Geometry check sheet. Reference: the model listing, model coordinates, mm. A direction names the side the tool comes from. Round coordinates to 2 decimals unless told otherwise and drop trailing zeros. Loops run counter-clockwise (first coordinate to the right, second up) from the corner with the lowest first, then second, coordinate; pieces in that order, holes last. Notation, with made-up numbers: (-3.75, 38) - (27.25, 38) arc R20 ccw to (27.25, 51) - close; hole circle Ø8 at (-2.5, 29). An arc over 180 degrees is marked (long way). Write item = value, one per line.
```python
from build123d import *

# Parameters (mm, degrees)
SKETCH1_W           = 156
SKETCH1_H           = 196
BASE_FLANGE1_DEPTH  = 0.5
EDGE_FLANGE1_DEPTH  = 196
EDGE_FLANGE2_DEPTH  = 156
EDGE_FLANGE3_DEPTH  = 196
EDGE_FLANGE4_DEPTH  = 156
SKETCH14_R          = 3
CUT_EXTRUDE1_DEPTH  = 2
CUT_EXTRUDE2_START  = -0.5
CUT_EXTRUDE2_DEPTH  = 0.5
CUT_EXTRUDE7_START  = -0.5
CUT_EXTRUDE7_DEPTH  = 0.5
SKETCH18_R          = 2
CUT_EXTRUDE8_DEPTH  = 254.83311453
SKETCH19_R          = 2
CUT_EXTRUDE9_DEPTH  = 255.06938035
SKETCH20_R          = 4
CUT_EXTRUDE10_DEPTH = 5
CUT_EXTRUDE11_START = -5
SKETCH21_R          = 4
CUT_EXTRUDE11_DEPTH = 5
SKETCH22_R          = 4
CUT_EXTRUDE12_DEPTH = 5
CUT_EXTRUDE13_START = -5
SKETCH23_R          = 4
CUT_EXTRUDE13_DEPTH = 5
SKETCH24_R          = 10
CUT_EXTRUDE14_DEPTH = 1
SKETCH25_R          = 2
CUT_EXTRUDE15_DEPTH = 2


# Read off the part's stored shape, not the designer's step: Cut-Extrude2, Cut-Extrude7
# Sheet-metal steps are written as plain solids
with BuildPart() as part:
    # Sketch1 → Base-Flange1 (new body)
    with BuildSketch(Plane(origin=(0, 0, 0), x_dir=(1, 0, 0), z_dir=(0, 1, 0))):
        with Locations((78, -98)):
            Rectangle(SKETCH1_W, SKETCH1_H)
    extrude(amount=-BASE_FLANGE1_DEPTH)

    # Edge-Flange1 section (across the edge) → Edge-Flange1 (add)
    with BuildSketch(Plane(origin=(-1, 0, 0), x_dir=(1, 0, 0), z_dir=(0, 0, 1))):
        with BuildLine():
            Line((-0.5, 1), (-0.5, 12))
            Line((-0.5, 12), (0, 12))
            Line((0, 12), (0, 1))
            ThreePointArc((0, 1), (0.292893219, 0.292893219), (1, 0))
            Line((1, 0), (1, -0.5))
            ThreePointArc((1, -0.5), (-0.060660172, -0.060660172), (-0.5, 1))
        make_face()
    extrude(amount=EDGE_FLANGE1_DEPTH)

    # Edge-Flange2 section (across the edge) → Edge-Flange2 (add)
    with BuildSketch(Plane(origin=(0, 0, 197), x_dir=(0, 0, -1), z_dir=(1, 0, 0))):
        with BuildLine():
            Line((-0.5, 1), (-0.5, 12))
            Line((-0.5, 12), (0, 12))
            Line((0, 12), (0, 1))
            ThreePointArc((0, 1), (0.292893219, 0.292893219), (1, 0))
            Line((1, 0), (1, -0.5))
            ThreePointArc((1, -0.5), (-0.060660172, -0.060660172), (-0.5, 1))
        make_face()
    extrude(amount=EDGE_FLANGE2_DEPTH)

    # Edge-Flange3 section (across the edge) → Edge-Flange3 (add)
    with BuildSketch(Plane(origin=(157, 0, 196), x_dir=(-1, 0, 0), z_dir=(0, 0, -1))):
        with BuildLine():
            Line((-0.5, 1), (-0.5, 12))
            Line((-0.5, 12), (0, 12))
            Line((0, 12), (0, 1))
            ThreePointArc((0, 1), (0.292893219, 0.292893219), (1, 0))
            Line((1, 0), (1, -0.5))
            ThreePointArc((1, -0.5), (-0.060660172, -0.060660172), (-0.5, 1))
        make_face()
    extrude(amount=EDGE_FLANGE3_DEPTH)

    # Edge-Flange4 section (across the edge) → Edge-Flange4 (add)
    with BuildSketch(Plane(origin=(156, 0, -1), x_dir=(0, 0, 1), z_dir=(-1, 0, 0))):
        with BuildLine():
            Line((-0.5, 1), (-0.5, 12))
            Line((-0.5, 12), (0, 12))
            Line((0, 12), (0, 1))
            ThreePointArc((0, 1), (0.292893219, 0.292893219), (1, 0))
            Line((1, 0), (1, -0.5))
            ThreePointArc((1, -0.5), (-0.060660172, -0.060660172), (-0.5, 1))
        make_face()
    extrude(amount=EDGE_FLANGE4_DEPTH)

    # Sketch14 → Cut-Extrude1 (cut)
    with BuildSketch(Plane.XY.offset(197.5)):
        with Locations((88.5, 5.312571767)):
            Circle(SKETCH14_R)
        with Locations((67.5, 5.312571767)):
            Circle(SKETCH14_R)
    extrude(amount=-CUT_EXTRUDE1_DEPTH, mode=Mode.SUBTRACT)

    # Cut-Extrude2 outline → Cut-Extrude2 (cut)
    with BuildSketch(Plane.ZY.offset(1.5).offset(CUT_EXTRUDE2_START)):
        with BuildLine():
            ThreePointArc((7.181368129, 12), (14.44892966, 4.034634629), (24.795691895, 1))
            add(Edge.make_bspline(
                [(24.795691895, 1), (24.960369193, 1), (25.12504649, 1), (25.289723788, 1)],
                knots=[0, 0, 0, 0, 1, 1, 1, 1], degree=3))
            ThreePointArc((25.289723788, 1), (35.636486024, 4.034634629), (42.904047554, 12))
            Line((42.904047554, 12), (7.181368129, 12))
        make_face()
        with BuildLine():
            Line((189.110571099, 12), (153.389428901, 12))
            ThreePointArc((153.389428901, 12), (171.25, 1), (189.110571099, 12))
        make_face()
    extrude(amount=CUT_EXTRUDE2_DEPTH, mode=Mode.SUBTRACT)

    # Cut-Extrude7 outline → Cut-Extrude7 (cut)
    with BuildSketch(Plane(origin=(157.5, 0, 0), x_dir=(0, 0, -1), z_dir=(1, 0, 0)).offset(CUT_EXTRUDE7_START)):
        with BuildLine():
            ThreePointArc((-189.110571099, 12), (-171.25, 1), (-153.389428901, 12))
            Line((-153.389428901, 12), (-189.110571099, 12))
        make_face()
        with BuildLine():
            add(Edge.make_bspline(
                [(-24.795691895, 1), (-24.960369193, 1), (-25.12504649, 1), (-25.289723788, 1)],
                knots=[0, 0, 0, 0, 1, 1, 1, 1], degree=3))
            ThreePointArc((-24.795691895, 1), (-14.44892966, 4.034634629), (-7.181368129, 12))
            Line((-7.181368129, 12), (-42.904047554, 12))
            ThreePointArc((-42.904047554, 12), (-35.636486024, 4.034634629), (-25.289723788, 1))
        make_face()
    extrude(amount=CUT_EXTRUDE7_DEPTH, mode=Mode.SUBTRACT)

    # Sketch18 → Cut-Extrude8 (cut, through all)
    with BuildSketch(Plane(origin=(157.5, 0, 0), x_dir=(0, 0, -1), z_dir=(1, 0, 0))):
        with Locations(Location((-98.146856175, 5.118141575, 0), (0, 0, 90))):
            Circle(SKETCH18_R)
    extrude(amount=-CUT_EXTRUDE8_DEPTH, mode=Mode.SUBTRACT)

    # Sketch19 → Cut-Extrude9 (cut, through all)
    with BuildSketch(Plane.XY.offset(197.5)):
        with Locations((27.98454493, 5.280354993)):
            Circle(SKETCH19_R)
        with Locations(Location((128.01545507, 5.280354993, 0), (0, 0, 180))):
            Circle(SKETCH19_R)
    extrude(amount=-CUT_EXTRUDE9_DEPTH, mode=Mode.SUBTRACT)

    # Sketch20 → Cut-Extrude10 (cut)
    with BuildSketch(Plane(origin=(157.5, 0, 0), x_dir=(0, 0, -1), z_dir=(1, 0, 0))):
        with Locations(Location((-88.146856175, 5.118141575, 0), (0, 0, 90))):
            Circle(SKETCH20_R)
        with Locations(Location((-108.146856175, 5.118141575, 0), (0, 0, 90))):
            Circle(SKETCH20_R)
    extrude(amount=-CUT_EXTRUDE10_DEPTH, mode=Mode.SUBTRACT)

    # Sketch21 → Cut-Extrude11 (cut)
    with BuildSketch(Plane.ZY.offset(1.5).offset(CUT_EXTRUDE11_START)):
        with Locations(Location((88.146856175, 5.118141575, 0), (0, 0, 90))):
            Circle(SKETCH21_R)
        with Locations(Location((108.146856175, 5.118141575, 0), (0, 0, 90))):
            Circle(SKETCH21_R)
    extrude(amount=CUT_EXTRUDE11_DEPTH, mode=Mode.SUBTRACT)

    # Sketch22 → Cut-Extrude12 (cut)
    with BuildSketch(Plane.XY.offset(197.5)):
        with Locations((138, 5.25)):
            Circle(SKETCH22_R)
        with Locations((118, 5.25)):
            Circle(SKETCH22_R)
        with Locations((38, 5.25)):
            Circle(SKETCH22_R)
        with Locations((18, 5.25)):
            Circle(SKETCH22_R)
    extrude(amount=-CUT_EXTRUDE12_DEPTH, mode=Mode.SUBTRACT)

    # Sketch23 → Cut-Extrude13 (cut)
    with BuildSketch(Plane(origin=(0, 0, -1.5), x_dir=(-1, 0, 0), z_dir=(0, 0, -1)).offset(CUT_EXTRUDE13_START)):
        with Locations(Location((-18, 5.25, 0), (0, 0, 180))):
            Circle(SKETCH23_R)
        with Locations(Location((-38, 5.25, 0), (0, 0, 180))):
            Circle(SKETCH23_R)
        with Locations(Location((-118, 5.25, 0), (0, 0, 180))):
            Circle(SKETCH23_R)
        with Locations(Location((-138, 5.25, 0), (0, 0, 180))):
            Circle(SKETCH23_R)
    extrude(amount=CUT_EXTRUDE13_DEPTH, mode=Mode.SUBTRACT)

    # Sketch24 → Cut-Extrude14 (cut)
    with BuildSketch(Plane.XY.offset(197.5)):
        with Locations((78, 17.812571767)):
            Circle(SKETCH24_R)
    extrude(amount=-CUT_EXTRUDE14_DEPTH, mode=Mode.SUBTRACT)

    # Sketch25 → Cut-Extrude15 (cut)
    with BuildSketch(Plane.XZ.offset(0.5)):
        with Locations(Location((78, 182.993325715, 0), (0, 0, 270))):
            Circle(SKETCH25_R)
    extrude(amount=-CUT_EXTRUDE15_DEPTH, mode=Mode.SUBTRACT)


solid = part.part
```
(1) Scan lines: L1, parallel to Z at x = 50.5, y = 4.75; L2, parallel to X at y = 2, z = 182; L3, parallel to Y at x = 87, z = 188. Record each from-to range of solid material in increasing order. Write a range as [from, to].
Answers follow:
L1 = [-1.5, -1], [197, 197.5]
L2 = [-1.5, -1], [157, 157.5]
L3 = [-0.5, 0]
(2) Gauge pin test, flat ends, axial feed: pin 1 (1.6 mm diameter, centred on x = -1, y = 4.5, fed in from +Z); pin 2 (5 mm diameter, centred on x = 65.5, z = 65, fed in from +Y). Record the tip position at first contact, or that the pin passes through.
Answers follow:
pin_1 = 196
pin_2 = 0
(3) Section check C-C (z = 74.5). Enter the section's corners in (x, y), then the cut area to 3 significant figures.
Answers follow:
outline = (-1.5, 1) arc R1.5 ccw to (0, -0.5) - (156, -0.5) arc R1.5 ccw to (157.5, 1) - (157.5, 12) - (157, 12) - (157, 1) arc R1 cw to (156, 0) - (0, 0) arc R1 cw to (-1, 1) - (-1, 12) - (-1.5, 12) - close
area = 91.0 mm²
(4) Section check D-D (x = 104). Enter the section's corners in (y, z).
Answers follow:
outline = (-0.5, 0) arc R1.5 ccw to (1, -1.5) - (12, -1.5) - (12, -1) - (1, -1) arc R1 cw to (0, 0) - (0, 196) arc R1 cw to (1, 197) - (12, 197) - (12, 197.5) - (1, 197.5) arc R1.5 ccw to (-0.5, 196) - close
(5) Section check A-A (x = 138). Enter the section's corners in (y, z).
Answers follow:
outline = (-0.5, 0) arc R1.5 ccw to (1, -1.5) - (1.25, -1.5) - (1.25, -1) - (1, -1) arc R1 cw to (0, 0) - (0, 196) arc R1 cw to (1, 197) - (1.25, 197) - (1.25, 197.5) - (1, 197.5) arc R1.5 ccw to (-0.5, 196) - close; (9.25, -1.5) - (12, -1.5) - (12, -1) - (9.25, -1) - close; (9.25, 197) - (12, 197) - (12, 197.5) - (9.25, 197.5) - close
(6) Mould release check, pull along X, two halves, no side actions. Record for faces 4 (the cylindrical face through (-1.25, 4.25, 92.05)), 5 (the flat face through (157.5, 8, 99)), 6 (the flat face through (157, 5, 189)): pulls with the +X half, pulls with the -X half, needs draft (parallel to the pull), parting line crosses it, or undercut.
Answers follow:
face_4 = needs draft
face_5 = pulls with the +X half
face_6 = undercut
(7) Set-up check for faces 1 (the cylindrical face through (-1.246, 4.116, 14.32)), 2 (the flat face through (-1, 8, 97)), 3 (the cylindrical face through (77.867, 7.813, 197.254)): record each of +Z, -Z, +X, -X, +Y, -Y from which the full face is reachable in a straight line by a thin tool's end or side.
Answers follow:
face_1 = +X, -X, +Y
face_2 = +Z, -Z, +Y
face_3 = +Z, +Y
(8) Section check B-B (x = 67.5). Enter the section's corners in (y, z).
Answers follow:
outline = (-0.5, 0) arc R1.5 ccw to (1, -1.5) - (12, -1.5) - (12, -1) - (1, -1) arc R1 cw to (0, 0) - (0, 196) arc R1 cw to (1, 197) - (2.31, 197) - (2.31, 197.5) - (1, 197.5) arc R1.5 ccw to (-0.5, 196) - close; (8.31, 197) - (12, 197) - (12, 197.5) - (8.31, 197.5) - close
